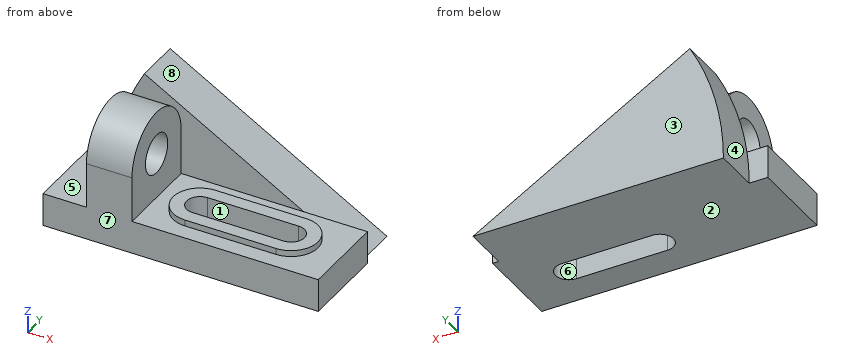
from build123d import *

# Parameters (mm, degrees)
F1_DEPTH = 42
F2_R     = 9.5
F3_DEPTH = 43.001
F5_DEPTH = 3
F7_DEPTH = 19.001
F9_DEPTH = 22


with BuildPart() as f1:
    # F0 (on Front) → F1 (new body)
    with BuildSketch(Plane.XZ):
        Polygon((0, 16), (0, 0), (133, 0), (133, 16), (43, 16), (43, 86), (21, 86), (21, 16), align=None)
    extrude(amount=F1_DEPTH)

    # F2 (on face) → F3 (cut, through all)
    with BuildSketch(Plane.YZ.offset(43)):
        with Locations((-21, 38)):
            Circle(F2_R)
        with BuildLine():
            Line((-42, 86), (-42, 38))
            ThreePointArc((-42, 38), (-21, 59), (0, 38))
            Line((0, 38), (0, 86))
            Line((0, 86), (-42, 86))
        make_face()
    extrude(amount=-F3_DEPTH, mode=Mode.SUBTRACT)

    # F4 (on face) → F5 (join)
    with BuildSketch(Plane.XY.offset(16)):
        with BuildLine():
            Line((108, -8), (64, -8))
            ThreePointArc((64, -8), (51, -21), (64, -34))
            Line((64, -34), (108, -34))
            ThreePointArc((108, -34), (121, -21), (108, -8))
        make_face()
    extrude(amount=F5_DEPTH)

    # F6 (on face) → F7 (cut, through all)
    with BuildSketch(Plane.XY.offset(19)):
        with BuildLine():
            Line((108, -14.5), (64, -14.5))
            ThreePointArc((64, -14.5), (57.5, -21), (64, -27.5))
            Line((64, -27.5), (108, -27.5))
            ThreePointArc((108, -27.5), (114.5, -21), (108, -14.5))
        make_face()
    extrude(amount=-F7_DEPTH, mode=Mode.SUBTRACT)

    # F8 (on face) → F9 (join)
    with BuildSketch(Plane(origin=(0, 0, 0), x_dir=(-1, 0, 0), z_dir=(0, 1, 0))):
        with BuildLine():
            Line((-25.210926, 60.5), (-130, 0))
            Line((-130, 0), (-9, 0))
            ThreePointArc((-9, 0), (-13.122975, 31.317104), (-25.210926, 60.5))
        make_face()
    extrude(amount=F9_DEPTH)


solid = f1.part
Verification items for the finished model (mm, model axes). Face numbers are marked on the shaded views. A direction names the side the tool comes from. Coordinates: 2 decimals unless noted, no trailing zeros. Write each loop counter-clockwise with the first axis right and the second up, starting at its lowest first coordinate (ties: lowest second). Pieces come first, ordered by that corner, then holes. Notation, with made-up numbers: M 61,-37 L 95,-37 A20 ccw 95,-8 Z; hole C 25.25,47.25 d10. An arc over 180 degrees is marked long. Use CSV: the item, a comma, the result in double quotes.
Q1. Thickness scan on line 1 along Z through (x, y) = (36, -21); line 2 along Y through (x, z) = (103, 18); line 3 along X through (y, z) = (-1.5, 31.5). Record the ranges inside material, lowest first. Write a range as [from, to].
Computed values:
line 1,"[0, 28.5], [47.5, 59]"
line 2,"[-34, -27.5], [-14.5, -8]"
line 3,"[21, 43]"
Q2. Mould release check, pull along Y, two halves, no side actions. Record for the marked faces 6, 7 and 8: pulls with the +Y half, pulls with the -Y half, needs draft (parallel to the pull), parting line crosses it, or undercut.
Computed values:
face 6,"undercut"
face 7,"pulls with the -Y half"
face 8,"needs draft"
Q3. Go/stop test with flat-tipped pins: P1, Ø1.5, axis at y = -19, z = 52, coming from the +X side; P2, Ø21, axis at y = -28, z = 44, coming from the -X side; P3, Ø13, axis at x = 81.5, y = -24.5, coming from the +Z side. Record where each tip stops, or that it passes through.
Computed values:
P1,"x = 43"
P2,"x = 21"
P3,"z = 19"
Q4. Section check D-D, the plane z = 13.5. Enter the section's corners in (x, y).
Computed values:
outline,"M 0,-42 L 133,-42 L 133,0 L 106.62,0 L 106.62,22 L 9.76,22 L 9.76,0 L 0,0 Z; hole M 64,-27.5 L 108,-27.5 A6.5 ccw 108,-14.5 L 64,-14.5 A6.5 ccw Z"
Q5. Set-up check for the marked faces 1, 2, 3, 4 and 5: record each of +Z, -Z, +X, -X, +Y, -Y from which the full face is reachable in a straight line by a thin tool's end or side.
Computed values:
face 1,"+Z, -Z"
face 2,"-Z, +X, -X, +Y, -Y"
face 3,"+Z, -Z, +X, -X, +Y"
face 4,"+Z, -X, +Y"
face 5,"+Z, -X, -Y"
Q6. Section check C-C, the plane z = 43.5. Enter the section's corners in (x, y).
Computed values:
outline,"M 17.09,0 L 54.66,0 L 54.66,22 L 17.09,22 Z; M 21,-41.27 L 43,-41.27 L 43,-28.75 L 21,-28.75 Z; M 21,-13.25 L 43,-13.25 L 43,-0.73 L 21,-0.73 Z"
Q7. Section check B-B, the plane x = 97.5. Enter the section's corners in (y, z).
Computed values:
outline,"M -42,0 L -27.5,0 L -27.5,19 L -34,19 L -34,16 L -42,16 Z; M -14.5,0 L 22,0 L 22,18.76 L 0,18.76 L 0,16 L -8,16 L -8,19 L -14.5,19 Z"
Q8. Section check A-A, the plane y = -21. Enter the section's corners in (x, z).
Computed values:
outline,"M 0,0 L 57.5,0 L 57.5,19 L 51,19 L 51,16 L 43,16 L 43,28.5 L 21,28.5 L 21,16 L 0,16 Z; M 21,47.5 L 43,47.5 L 43,59 L 21,59 Z; M 114.5,0 L 133,0 L 133,16 L 121,16 L 121,19 L 114.5,19 Z"
